from build123d import *

# Parameters (mm, degrees)
SKETCH2_R               = 60
BOSS_EXTRUDE1_DEPTH     = 360
SKETCH3_R               = 70
BOSS_EXTRUDE2_DEPTH     = 10
BOSS_EXTRUDE4_DEPTH     = 8
BOSS_EXTRUDE5_DEPTH     = 5
CIRPATTERN1_COUNT       = 4
SKETCH5_R               = 8.25
CUT_EXTRUDE2_DEPTH      = 10
SKETCH8_R               = 8.25
CUT_EXTRUDE3_DEPTH      = 10
CUT_EXTRUDE8_DEPTH      = 25
CUT_EXTRUDE8_DEPTH_BACK = 22
SKETCH9_R               = 4.4


with BuildPart() as part:
    # Sketch2 → Boss-Extrude1 (new body)
    with BuildSketch(Plane.XY):
        Circle(SKETCH2_R)
    extrude(amount=BOSS_EXTRUDE1_DEPTH)

    # Sketch3 → Boss-Extrude2 (add)
    with BuildSketch(Plane(origin=(0, 0, 0), x_dir=(-1, 0, 0), z_dir=(0, 0, -1))):
        Circle(SKETCH3_R)
    extrude(amount=BOSS_EXTRUDE2_DEPTH)

    # Sketch4 → Boss-Extrude4 (add)
    with BuildSketch(Plane.XY.offset(360)):
        Polygon((-70, 120), (-120, 70), (-120, -70), (-70, -120), (70, -120), (120, -70), (120, 70), (70, 120), align=None)
    extrude(amount=BOSS_EXTRUDE4_DEPTH)

    # Sketch7 → Boss-Extrude5 (add, symmetric)
    with BuildSketch(Plane(origin=(0, 0, 0), x_dir=(0, 0, -1), z_dir=(1, 0, 0))):
        Polygon((-360, -120), (-260, -55), (-360, -55), align=None)
    boss_extrude5 = extrude(amount=BOSS_EXTRUDE5_DEPTH, both=True)

    # CirPattern1: Boss-Extrude5 ×4 about axis
    cirpattern1_axis = Axis((0, 0, 0), (0, 0, 1))
    for i in range(1, CIRPATTERN1_COUNT):
        add(boss_extrude5.rotate(cirpattern1_axis, i * 360 / CIRPATTERN1_COUNT))

    # Sketch5 → Cut-Extrude2 (cut)
    with BuildSketch(Plane.XY.offset(368)):
        with Locations((-39.145715053, 95)):
            Circle(SKETCH5_R)
        with Locations((-39.145715053, -95)):
            Circle(SKETCH5_R)
        with Locations((49.020413154, 95)):
            Circle(SKETCH5_R)
        with Locations((49.020413154, -95)):
            Circle(SKETCH5_R)
    extrude(amount=-CUT_EXTRUDE2_DEPTH, mode=Mode.SUBTRACT)

    # Sketch8 → Cut-Extrude3 (cut)
    with BuildSketch(Plane.XY.offset(368)):
        with Locations((-86.808078285, 65.641177005)):
            Circle(SKETCH8_R)
        with Locations((-86.808078285, -55.652302243)):
            Circle(SKETCH8_R)
        with Locations((94.418649532, -55.652302243)):
            Circle(SKETCH8_R)
        with Locations((88.710721097, 59.457587867)):
            Circle(SKETCH8_R)
    extrude(amount=-CUT_EXTRUDE3_DEPTH, mode=Mode.SUBTRACT)

    # Sketch9 → Cut-Extrude8 (cut, two sides: drawn at the far end of the back side and taken through both)
    with BuildSketch(Plane(origin=(0, 0, -10), x_dir=(-1, 0, 0), z_dir=(0, 0, -1)).offset(-CUT_EXTRUDE8_DEPTH_BACK)):
        with Locations(Location((0, 63.204671138, 0), (0, 0, 228.131406789))):
            Circle(SKETCH9_R)
        with Locations((1.290982991, -53.670475155)):
            Circle(SKETCH9_R)
        with Locations(Location((53.562270393, 32.283588378, 0), (0, 0, 157.987594356))):
            Circle(SKETCH9_R)
        with Locations(Location((-50.426550115, 34.101651925, 0), (0, 0, 249.437866914))):
            Circle(SKETCH9_R)
        with Locations(Location((52.769279557, -32.934214303, 0), (0, 0, 206.210166052))):
            Circle(SKETCH9_R)
        with Locations(Location((-51.084491131, -34.716860238, 0), (0, 0, 98.670706964))):
            Circle(SKETCH9_R)
    extrude(amount=CUT_EXTRUDE8_DEPTH + CUT_EXTRUDE8_DEPTH_BACK, mode=Mode.SUBTRACT)


solid = part.part
Geometry check sheet. Reference: the model listing, model coordinates, mm. A direction names the side the tool comes from. Give positions to 0.01 mm unless a question says otherwise; leave off trailing zeros. Order: outer loops, then holes, each group sorted by start corner. A loop starts at its lowest first (then second) coordinate and runs counter-clockwise, first axis right, second up.
1) Gauge pin test, flat ends, axial feed: pin 1 (3 mm diameter, centred on x = 2, z = 269, fed in from +Y) (3 decimals); pin 2 (6 mm diameter, centred on y = -89.5, z = 312, fed in from -X); pin 3 (1 mm diameter, centred on x = -54.5, z = 148.5, fed in from +Y); pin 4 (19 mm diameter, centred on x = 94.42, y = -55.65, fed in from +Z). Record the tip position at first contact, or that the pin passes through.
Results are:
pin 1: stops at y = 61.825
pin 2: stops at x = -5
pin 3: stops at y = 26.15
pin 4: stops at z = 368
2) Tool access check on faces 4 (the cylindrical face through (55.425, -22.98, 177.48)), 5 (the cylindrical face through (-0.718, -49.308, 1.154)), 6 (the flat face through (-1, -120, 364)). Record the directions out of +Z, -Z, +X, -X, +Y, -Y that give a thin tool (end or side, any length) a straight path to the whole face; none if there is none.
Results are:
face 4: none
face 5: -Z
face 6: +Z, -Z, +X, -X, -Y
3) Cross-section at B-B (z = 314). Record the boundary of the cut face in (x, y), then the cut area to 3 significant figures.
Results are:
outline: (-90.1, -5) - (-59.79, -5) arc R60 ccw to (-5, -59.79) - (-5, -90.1) - (5, -90.1) - (5, -59.79) arc R60 ccw to (59.79, -5) - (90.1, -5) - (90.1, 5) - (59.79, 5) arc R60 ccw to (5, 59.79) - (5, 90.1) - (-5, 90.1) - (-5, 59.79) arc R60 ccw to (-59.79, 5) - (-90.1, 5) - close
area: 12,500 mm2
4) Cross-section at D-D (y = 0). Record the boundary of the cut face in (x, z), then the cut area to 3 significant figures.
Results are:
outline: (-120, 360) - (-60, 267.69) - (-60, 0) - (-70, 0) - (-70, -10) - (70, -10) - (70, 0) - (60, 0) - (60, 267.69) - (120, 360) - (120, 368) - (-120, 368) - close
area: 52,100 mm2
5) Cross-section at C-C (x = 21.5). Record the boundary of the cut face in (y, z).
Results are:
outline: (-120, 360) - (-56.02, 360) - (-56.02, 0) - (-66.62, 0) - (-66.62, -10) - (66.62, -10) - (66.62, 0) - (56.02, 0) - (56.02, 360) - (120, 360) - (120, 368) - (-120, 368) - close
6) Cross-section at A-A (y = -95). Record the boundary of the cut face in (x, z), then the cut area to 3 significant figures.
Results are:
outline: (-95, 360) - (-47.4, 360) - (-47.4, 368) - (-95, 368) - close; (-30.9, 360) - (-5, 360) - (-5, 321.54) - (5, 321.54) - (5, 360) - (40.77, 360) - (40.77, 368) - (-30.9, 368) - close; (57.27, 360) - (95, 360) - (95, 368) - (57.27, 368) - close
area: 1,640 mm2
7) Draft check along Y on faces 1 (the flat face through (1, 120, 364)), 2 (the cylindrical face through (-1.184, 58.967, -3.735)), 3 (the flat face through (1, 1, -10)). Enter one of: released by +Y, released by -Y, zero draft, split by the parting line, or undercut.
Results are:
face 1: released by +Y
face 2: undercut
face 3: zero draft
8) Material ranges on probe 1 along Z at (x, y) = (58, 27.5); probe 2 along Z at (x, y) = (-89, 30.5); probe 3 along X at (y, z) = (-90, 348), recorded low to high.
Results are:
probe 1: z = -10 to 0, 360 to 368
probe 2: z = 360 to 368
probe 3: x = -5 to 5
